from build123d import *

# Parameters (mm, degrees)
F0_R           = 7
F0_R_2         = 6
F1_DEPTH       = 12
F0_R_3         = 5
F2_DEPTH       = 24
F3_DEPTH       = 24
F3_DEPTH_BACK  = 12
F4_SIZE        = 1
F5_SIZE        = 0.5
F6_R           = 3
F7_DEPTH       = 25
F7_DEPTH_BACK  = 25
F9_R           = 6
F10_DEPTH      = 26
F10_DEPTH_BACK = 40
F11_SIZE       = 1
F12_DEPTH      = 25
F12_DEPTH_BACK = 25
F13_R          = 2.5
F14_DEPTH      = 15


with BuildPart() as f1:
    # F0 (on Front) → F1 (new body)
    with BuildSketch(Plane.XZ):
        Circle(F0_R)
        Circle(F0_R_2, mode=Mode.SUBTRACT)
    extrude(amount=F1_DEPTH)

    # F0 (on Front) → F2 (join)
    with BuildSketch(Plane.XZ):
        Circle(F0_R_2)
        Circle(F0_R_3, mode=Mode.SUBTRACT)
    extrude(amount=F2_DEPTH)

    # F0 (on Front) → F3 (join, two sides)
    with BuildSketch(Plane.XZ) as f3_sk:
        Circle(F0_R_3)
    extrude(amount=F3_DEPTH)
    extrude(f3_sk.sketch, amount=-F3_DEPTH_BACK)

    # F4
    f4_edges = [f1.edges().sort_by_distance(p)[0] for p in [
        (-5, 12, 0),
    ]]
    chamfer(f4_edges, length=F4_SIZE)

    # F5
    f5_edges = [f1.edges().sort_by_distance(p)[0] for p in [
        (-6, -24, 0),
        (-7, -12, 0),
        (7, -6, 0),
        (-7, 0, 0),
    ]]
    chamfer(f5_edges, length=F5_SIZE)

    # F6 (on Top) → F7 (cut, two sides)
    with BuildSketch(Plane.XY) as f7_sk:
        with Locations((0, -18)):
            Circle(F6_R)
        with Locations((0, -78)):
            Circle(F6_R)
    extrude(amount=-F7_DEPTH, mode=Mode.SUBTRACT)
    extrude(f7_sk.sketch, amount=F7_DEPTH_BACK, mode=Mode.SUBTRACT)

    # F9 (on offset) → F10 (join, two sides)
    with BuildSketch(Plane.XZ.offset(49)) as f10_sk:
        Circle(F9_R)
    extrude(amount=-F10_DEPTH)
    extrude(f10_sk.sketch, amount=F10_DEPTH_BACK)

    # F11
    f11_edges = [f1.edges().sort_by_distance(p)[0] for p in [
        (-6, -89, 0),
    ]]
    chamfer(f11_edges, length=F11_SIZE)

    # F6 (on Top) → F12 (cut, two sides)
    with BuildSketch(Plane.XY) as f12_sk:
        with Locations((0, -18)):
            Circle(F6_R)
        with Locations((0, -78)):
            Circle(F6_R)
    extrude(amount=F12_DEPTH, mode=Mode.SUBTRACT)
    extrude(f12_sk.sketch, amount=-F12_DEPTH_BACK, mode=Mode.SUBTRACT)

    # F13 (on face) → F14 (cut)
    with BuildSketch(Plane.XZ.offset(89)):
        Circle(F13_R)
    extrude(amount=-F14_DEPTH, mode=Mode.SUBTRACT)


solid = f1.part
Verification items for the finished model (mm, model axes). A direction names the side the tool comes from. Round coordinates to 2 decimals unless told otherwise and drop trailing zeros. Loops run counter-clockwise (first coordinate to the right, second up) from the corner with the lowest first, then second, coordinate; pieces in that order, holes last. Notation, with made-up numbers: (-35, 40) - (-26, 40) arc R8 cw to (-26, 44) - close; hole circle Ø3 at (57.25, -27.75). An arc over 180 degrees is marked (long way). Use a Markdown table: item, result. Add a question column.
1. Section check D-D, the plane y = -14. Record the boundary of the cut face in (x, z).
2. Section check A-A, the plane x = -1.5. Give the number of separate pieces and of enclosed holes in the cut face, plus the area to 3 significant figures.
3. Thickness scan on probe 1 along Y at (x, z) = (0, 4); probe 2 along Y at (x, z) = (0, 1.5); probe 3 along Y at (x, z) = (0.75, 4.5). Record the ranges inside material, lowest first. Write a range as [from, to].
4. Section check B-B, the plane y = 1.5. Record the boundary of the cut face in (x, z), plus the area to 3 significant figures.
5. Section check C-C, the plane y = -78. Record the boundary of the cut face in (x, z).
6. Release check for a two-part mould opening along Z. For faces 1 (the face through (-2, -74.9, -1.5)), 2 (the face through (2, -12, -6)), 3 (the face through (2.31, -84.39, -0.96)), 4 (the face through (-1.08, 5.42, -4.88)) record: released by +Z, released by -Z, zero draft, split by the parting line, or undercut.
7. Gauge pin test, flat ends, axial feed: pin 1 (2 mm diameter, centred on x = -4.5, y = -67.5, fed in from +Z); pin 2 (1.5 mm diameter, centred on x = 4, z = -5, fed in from +Y); pin 3 (3 mm diameter, centred on x = -3, y = -27.5, fed in from -Z). Record the tip position at first contact, or that the pin passes through.
8. Access from +Z, -Z, +X, -X, +Y, -Y to the whole of each face (thin tool, end or side, straight path). Record for faces 5 (the face through (2, 0, -5)), 6 (the face through (0, -74, 0)), 7 (the face through (6.466, -5.923, -2.681)).
Checks:
| question | item | result |
|---|---|---|
| 1 | outline | circle Ø12 at (0, 0) |
| 2 | separate pieces | 4 |
| 2 | enclosed holes | 0 |
| 2 | area | 1,010 mm^2 |
| 3 | probe 1 | y = [-89, -81], [-75, -21], [-15, 12] |
| 3 | probe 2 | y = [-74, -21], [-15, 12] |
| 3 | probe 3 | y = [-89, -80.9], [-75.1, -20.9], [-15.1, 11.44] |
| 4 | outline | circle Ø10 at (0, 0) |
| 4 | area | 78.5 mm^2 |
| 5 | outline | (-3, -5.2) - (-3, 5.2) arc R6 ccw to start; (3, -5.2) arc R6 ccw to (3, 5.2) - close |
| 6 | face 1 | undercut |
| 6 | face 2 | zero draft |
| 6 | face 3 | undercut |
| 6 | face 4 | split by the parting line |
| 7 | pin 1 | stops at z = 4.87 |
| 7 | pin 2 | stops at y = 0 |
| 7 | pin 3 | stops at z = -5.81 |
| 8 | face 5 | +Y |
| 8 | face 6 | -Y |
| 8 | face 7 | +Y, -Y |
